Can you work these out from the model? Positions are in its coordinate system, mm. A direction names the side the tool comes from. Round coordinates to 2 decimals unless told otherwise and drop trailing zeros. Order: outer loops, then holes, each group sorted by start corner. A loop starts at its lowest first (then second) coordinate and runs counter-clockwise, first axis right, second up. Notation, with made-up numbers: (22.5, 40) -> (58.5, 40) arc R21 cw to (58.5, 61) -> close; hole circle Ø4 at (14.5, -34.75). An arc over 180 degrees is marked (long way). One line per item, written item: value.
```python
from build123d import *

# Parameters (mm, degrees)
SKETCH_W     = 30
SKETCH_H     = 27.5
PAD_DEPTH    = 5
PAD001_DEPTH = 25
SKETCH002_W  = 15
SKETCH002_H  = 15
POCKET_DEPTH = 27.5
FILLET_R     = 2


with BuildPart() as part:
    # Sketch → Pad (new body)
    with BuildSketch(Plane.XY):
        with Locations((2.5, 0)):
            Rectangle(SKETCH_W, SKETCH_H)
    extrude(amount=-PAD_DEPTH)

    # Sketch001 → Pad001 (join)
    with BuildSketch(Plane.XY):
        Polygon((-12.5, 8.75), (12.5, 8.75), (12.5, -8.75), (-12.5, -8.75), (-12.5, -13.75), (17.5, -13.75), (17.5, 13.75), (-12.5, 13.75), align=None)
    extrude(amount=PAD001_DEPTH)

    # Sketch002 (on Face2 of Pad001) → Pocket (cut)
    with BuildSketch(Plane.XZ.offset(13.75)):
        with Locations((-5, 17.5)):
            Rectangle(SKETCH002_W, SKETCH002_H)
    extrude(amount=-POCKET_DEPTH, mode=Mode.SUBTRACT)

    # Fillet
    fillet_edges = [part.edges().sort_by_distance(p)[0] for p in [
        (2.5, 11.25, 25),
        (2.5, 11.25, 10),
        (-12.5, 11.25, 10),
        (2.5, -11.25, 25),
        (2.5, -11.25, 10),
        (-12.5, -11.25, 10),
        (17.5, 0, 25),
        (-12.5, 0, -5),
        (17.5, 0, -5),
        (17.5, 13.75, 10),
        (2.5, 13.75, -5),
        (10, -13.75, 25),
        (2.5, -13.75, -5),
        (17.5, -13.75, 10),
    ]]
    fillet(fillet_edges, radius=FILLET_R)


solid = part.part
```
Q1. I want a section at A-A on y = 6.5. List the corners of the cut face in (x, z) for me, plus the area to 3 significant figures.
Answers below:
outline: (-12.5, -3) arc R2 ccw to (-10.5, -5) -> (15.5, -5) arc R2 ccw to (17.5, -3) -> (17.5, 23) arc R2 ccw to (15.5, 25) -> (12.5, 25) -> (12.5, 0) -> (-12.5, 0) -> close
area: 272 mm^2
Q2. Will these pins go through, and if not, where does the flat tip stop? pin 1 Ø4 at (y, z) = (-4.5, 14) entering from -X; pin 2 Ø2.5 at (y, z) = (-10, 16) entering from -X; pin 3 Ø1.5 at (x, y) = (-4.5, 12) entering from +Z.
Answers below:
pin 1: x = 12.5
pin 2: x = 2.5
pin 3: z = 10
Q3. On a 3-axis mill with a long thin cutter (end or side, diameter ignored), from which of +Z, -Z, +X, -X, +Y, -Y can I reach the whole of each face in a straight line? I mean faces 1 (the face through (2.5, 11, 17)), 2 (the face through (12.5, 0, 12)), 3 (the face through (4, -13.75, 7)). Say none if no direction works.
Answers below:
face 1: +Z, -X, +Y, -Y
face 2: +Z, -X
face 3: +Z, -Z, +X, -X, -Y
Q4. Please list where these lines run through material, in increasing order: line 1 along Y through (x, z) = (3.75, 3); line 2 along X through (y, z) = (2, 20.25); line 3 along Z through (x, y) = (-9, 11.75).
Answers below:
line 1: -13.75 to -8.75, 8.75 to 13.75
line 2: 12.5 to 17.5
line 3: -5 to 10
Q5. I want a section at D-D on z = 6.25. List the corners of the cut face in (x, y) for me, plus the area to 3 significant figures.
Answers below:
outline: (-12.5, -13.75) -> (15.5, -13.75) arc R2 ccw to (17.5, -11.75) -> (17.5, 11.75) arc R2 ccw to (15.5, 13.75) -> (-12.5, 13.75) -> (-12.5, 8.75) -> (12.5, 8.75) -> (12.5, -8.75) -> (-12.5, -8.75) -> close
area: 386 mm^2
Q6. I want a section at B-B on z = 20.5. List the corners of the cut face in (x, y) for me.
Answers below:
outline: (2.5, -13.75) -> (15.5, -13.75) arc R2 ccw to (17.5, -11.75) -> (17.5, 11.75) arc R2 ccw to (15.5, 13.75) -> (2.5, 13.75) -> (2.5, 8.75) -> (12.5, 8.75) -> (12.5, -8.75) -> (2.5, -8.75) -> close
Q7. I want a section at C-C on x = 8.75. List the corners of the cut face in (y, z) for me.
Answers below:
outline: (-13.75, -3) arc R2 ccw to (-11.75, -5) -> (11.75, -5) arc R2 ccw to (13.75, -3) -> (13.75, 25) -> (8.75, 25) -> (8.75, 0) -> (-8.75, 0) -> (-8.75, 25) -> (-11.75, 25) arc R2 ccw to (-13.75, 23) -> close
